The listing builds one solid part. Answer for the finished solid, in the listing's coordinates (mm). A direction names the side the tool comes from. Give positions to 0.01 mm unless a question says otherwise; leave off trailing zeros. Order: outer loops, then holes, each group sorted by start corner. A loop starts at its lowest first (then second) coordinate and runs counter-clockwise, first axis right, second up.
```python
from build123d import *

# Parameters (mm, degrees)
SKETCH1_R           = 4.25
SKETCH1_R_2         = 0.55
BOSS_EXTRUDE1_DEPTH = 1
SKETCH2_R           = 1.5
BOSS_EXTRUDE2_DEPTH = 1.5
SKETCH3_R           = 5
BOSS_EXTRUDE3_DEPTH = 5
SKETCH4_R           = 0.5
BOSS_EXTRUDE4_DEPTH = 5
SKETCH5_R           = 0.75
CUT_EXTRUDE1_DEPTH  = 2
CHAMFER1_SIZE       = 0.5


with BuildPart() as part:
    # Sketch1 → Boss-Extrude1 (new body)
    with BuildSketch(Plane.XY):
        Circle(SKETCH1_R)
        with Locations((0, 3.3)):
            Circle(SKETCH1_R_2, mode=Mode.SUBTRACT)
        with Locations((2.857883832, -1.65)):
            Circle(SKETCH1_R_2, mode=Mode.SUBTRACT)
        with Locations((-2.857883832, -1.65)):
            Circle(SKETCH1_R_2, mode=Mode.SUBTRACT)
    extrude(amount=BOSS_EXTRUDE1_DEPTH)

    # Sketch2 → Boss-Extrude2 (add)
    with BuildSketch(Plane.XY.offset(1)):
        Circle(SKETCH2_R)
    extrude(amount=BOSS_EXTRUDE2_DEPTH)

    # Sketch3 → Boss-Extrude3 (add)
    with BuildSketch(Plane.XY.offset(2.5)):
        Circle(SKETCH3_R)
    extrude(amount=BOSS_EXTRUDE3_DEPTH)

    # Sketch4 → Boss-Extrude4 (add)
    with BuildSketch(Plane.XY.offset(7.5)):
        Circle(SKETCH4_R)
    extrude(amount=BOSS_EXTRUDE4_DEPTH)

    # Sketch5 → Cut-Extrude1 (cut)
    with BuildSketch(Plane.XY.offset(7.5)):
        with Locations((0, 3)):
            Circle(SKETCH5_R)
        with Locations((2.853169549, 0.927050983)):
            Circle(SKETCH5_R)
        with Locations((1.763355757, -2.427050983)):
            Circle(SKETCH5_R)
        with Locations((-1.763355757, -2.427050983)):
            Circle(SKETCH5_R)
        with Locations((-2.853169549, 0.927050983)):
            Circle(SKETCH5_R)
    extrude(amount=-CUT_EXTRUDE1_DEPTH, mode=Mode.SUBTRACT)

    # Chamfer1
    chamfer1_edges = [part.edges().sort_by_distance(p)[0] for p in [
        (-5, 0, 7.5),
    ]]
    chamfer(chamfer1_edges, length=CHAMFER1_SIZE)


solid = part.part
```
1) Find section A-A (y = 0). Write down the section's boundary in (x, z), then the cut area to 4 significant figures.
Geometry says:
outline: (-5, 2.5) - (-1.5, 2.5) - (-1.5, 1) - (-4.25, 1) - (-4.25, 0) - (4.25, 0) - (4.25, 1) - (1.5, 1) - (1.5, 2.5) - (5, 2.5) - (5, 7) - (4.5, 7.5) - (0.5, 7.5) - (0.5, 12.5) - (-0.5, 12.5) - (-0.5, 7.5) - (-4.5, 7.5) - (-5, 7) - close
area: 67.75 mm2
2) Find section B-B (z = 2). Write down the section's boundary in (x, y), then the cut area to 3 significant figures.
Geometry says:
outline: circle Ø3 at (0, 0)
area: 7.07 mm2
3) Straight lines are drawn through the part: probe 1 along Z at (x, y) = (1.25, 1.25); probe 2 along Y at (x, z) = (0, 0.75); probe 3 along Z at (x, y) = (2.25, -2.75). For each, find the intervals that lie inside material, in ascending order.
Geometry says:
probe 1: z = 0 to 1, 2.5 to 7.5
probe 2: y = -4.25 to 2.75, 3.85 to 4.25
probe 3: z = 0 to 1, 2.5 to 5.5
4) For a pull along X with two mould halves and no side action, classify faces 1 (the flat face through (0, 0, 12.5)), 2 (the cylindrical face through (-1.5, 0.07, 1.74)), 3 (the flat face through (0, 3, 5.5)) as +X half, -X half, draft (parallel to the pull), parting line (faces both ways), or undercut.
Geometry says:
face 1: draft
face 2: parting line
face 3: undercut
5) Given P1, Ø1.5, axis at y = 2, z = 9, coming from the +X side; P2, Ø1, axis at x = -4, z = 3, coming from the +Y side; P3, Ø1.8, axis at x = -2.86, y = -1.65, coming from the +Z side; P4, Ø0.8, axis at x = 0, y = 3, coming from the +Z side, each flat-ended and moving along its own axis, determine where each tip first touches the part or whether it passes through.
Geometry says:
P1: passes through
P2: stops at y = 3.57
P3: stops at z = 7.5
P4: stops at z = 5.5
6) A tool of negligible diameter and unlimited length cuts with its end or side. For faces 4 (the cylindrical face through (-3.294, -1.985, 0.493)), 5 (the flat face through (0, -2, 1)), 6 (the cylindrical face through (2.691, 0.195, 6.514)), from which of +Z, -Z, +X, -X, +Y, -Y can it reach the whole face along a straight path? Write none if from no direction.
Geometry says:
face 4: -Z
face 5: none
face 6: +Z
7) Find section C-C (x = 3.25). Count the separate pieces of the cut face and the enclosed holes in it, then the cut area to 3 significant figures.
Geometry says:
separate pieces: 3
enclosed holes: 0
area: 39.8 mm2
